Model file for the job. Use its own axes, mm. Face numbers are marked on the shaded views. A direction names the side the tool comes from. Round coordinates to 2 decimals unless told otherwise and drop trailing zeros. Order: outer loops, then holes, each group sorted by start corner. A loop starts at its lowest first (then second) coordinate and runs counter-clockwise, first axis right, second up. Notation, with made-up numbers: M 32,71.5 L 71,71.5 A32 ccw 71,99.5 Z; hole C 13,-31 d1. An arc over 180 degrees is marked long. Return JSON: item names as keys, results as strings. Group by question number.
Item 1: Pull direction X, two halves, no side cores. Call the marked faces 4, 5 and 6: pulls with the +X half, pulls with the -X half, needs draft (parallel to the pull), parting line crosses it, or undercut.
Item 2: Probe line 1 along X through (y, z) = (0, 4.75) (3 decimals); line 2 along Z through (x, y) = (5.5, 17.5). List the from-to ranges inside material, lowest first.
Item 3: Slice it at B-B on y = -10.5. Write the cut outline in (x, z), then the cut area to 3 significant figures.
Item 4: Slice it at C-C on z = 2.25. Write the cut outline in (x, y) (3 decimals).
Item 5: Slice it at A-A on x = 0. Write the cut outline in (y, z) (3 decimals), then the cut area to 3 significant figures.
Item 6: Slice it at D-D on y = -15. Write the cut outline in (x, z), then the cut area to 3 significant figures.
Item 7: Which spindle directions (+Z, -Z, +X, -X, +Y, -Y) get a long thin tool onto all of the face, cutting with end or side? Do the marked faces 1, 2 and 3. Say none if no direction does.
Item 8: Pin check, flat tips, straight feed: pin 1 Ø19 at (x, y) = (3, -1.5) entering from -Z; pin 2 Ø1 at (y, z) = (-9, 5.5) entering from -X; pin 3 Ø1.5 at (x, y) = (2.5, 15.5) entering from +Z. Stop position of each tip, or through.
from build123d import *

# Parameters (mm, degrees)
F0_R     = 22.225
F1_DEPTH = 12.7
F2_R     = 19.177
F3_DEPTH = 6.35
F4_R     = 4.05
F5_DEPTH = 22.226
F6_DEPTH = 12.7


with BuildPart() as f1:
    # F0 (on Top) → F1 (new body)
    with BuildSketch(Plane.XY):
        Circle(F0_R)
    extrude(amount=F1_DEPTH)

    # F2 (on face) → F3 (cut)
    with BuildSketch(Plane(origin=(0, 0, 0), x_dir=(1, 0, 0), z_dir=(0, 0, -1))):
        Circle(F2_R)
    extrude(amount=-F3_DEPTH, mode=Mode.SUBTRACT)

    # F4 (on Front) → F5 (cut, through all)
    with BuildSketch(Plane.XZ):
        with Locations((0, 12.7)):
            Circle(F4_R)
    extrude(amount=-F5_DEPTH, mode=Mode.SUBTRACT)

    # F4 (on Front) → F6 (cut)
    with BuildSketch(Plane.XZ):
        with Locations((0, 12.7)):
            Circle(F4_R)
    extrude(amount=F6_DEPTH, mode=Mode.SUBTRACT)


solid = f1.part
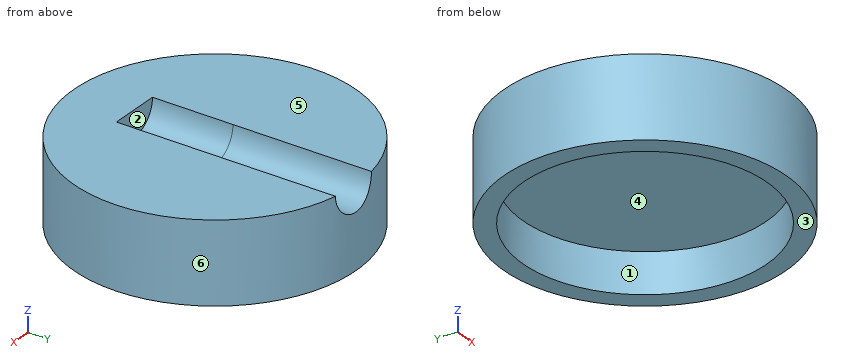
Output values:
{
 "1": {"face 4": "undercut", "face 5": "needs draft", "face 6": "parting line crosses it"},
 "2": {"line 1": "-22.225 to -19.177, 19.177 to 22.225", "line 2": "6.35 to 12.7"},
 "3": {"outline": "M -19.59,0 L -16.05,0 L -16.05,6.35 L 16.05,6.35 L 16.05,0 L 19.59,0 L 19.59,12.7 L 4.05,12.7 A4.05 cw -4.05,12.7 L -19.59,12.7 Z", "area": "268 mm²"},
 "4": {"outline": "C 0,0 d44.45; hole C 0,0 d38.354"},
 "5": {"outline": "M -22.225,0 L -19.177,0 L -19.177,6.35 L 19.177,6.35 L 19.177,0 L 22.225,0 L 22.225,8.65 L -12.7,8.65 L -12.7,12.7 L -22.225,12.7 Z", "area": "180 mm²"},
 "6": {"outline": "M -16.4,0 L -11.95,0 L -11.95,6.35 L 11.95,6.35 L 11.95,0 L 16.4,0 L 16.4,12.7 L -16.4,12.7 Z", "area": "265 mm²"},
 "7": {"face 1": "-Z", "face 2": "+Z, +Y", "face 3": "-Z, +X, -X, +Y, -Y"},
 "8": {"pin 1": "z = 6.35", "pin 2": "x = -20.54", "pin 3": "z = 10.28"}
}
